Source: CAD feature listing. Evaluate the final solid. Frame: model axes, mm. A direction names the side the tool comes from. Round coordinates to 2 decimals unless told otherwise and drop trailing zeros. Order: outer loops, then holes, each group sorted by start corner. A loop starts at its lowest first (then second) coordinate and runs counter-clockwise, first axis right, second up. Notation, with made-up numbers: (29, 59) -> (68, 59) arc R8 cw to (68, 65) -> close; hole circle Ø10 at (41, 85). An arc over 180 degrees is marked (long way). Write item = value, one per line. Start each with the question number.
(1) Reachability of faces 1 (the face through (13, 2, -26)), 2 (the face through (10, 2, -6)), 3 (the face through (10, 2, -10)) from +Z, -Z, +X, -X, +Y, -Y: full face, straight path, thin tool, end or side. Return the list, or none.
(2) Ray query, line 1 (X direction, y = 1.6, z = -25.25); line 2 (X direction, y = 2.85, z = -17); line 3 (Z direction, x = 9.5, y = 1.35). Return the intervals inside material, ascending.
(3) Cut plane A-A on z = -14.5. Return the cut outline in (x, y), then the cut area to 3 significant figures.
(4) Draft query along X for faces 4 (the face through (16, 2, 0)), 5 (the face through (13, 2, -3)), 6 (the face through (12.703, 2, -16)), 7 (the face through (0, 2, -14)). Return one class per face: released by +X, released by -X, zero draft, split by the parting line, or undercut.
(5) Cut plane B-B on y = 3.05. Return the cut outline in (x, z), then the cut area to 3 significant figures.
from build123d import *

# Parameters (mm, degrees)
SKETCH1_W           = 20
SKETCH1_H           = 28
BOSS_EXTRUDE1_DEPTH = 3.5
SKETCH2_W           = 6
SKETCH2_H           = 4.75
SKETCH2_H_2         = 6
CUT_EXTRUDE1_DEPTH  = 4.5
CUT_EXTRUDE6_DEPTH  = 4.5


with BuildPart() as part:
    # Sketch1 → Boss-Extrude1 (new body)
    with BuildSketch(Plane(origin=(0, 0, 0), x_dir=(1, 0, 0), z_dir=(0, 1, 0))):
        with Locations((10, 14)):
            Rectangle(SKETCH1_W, SKETCH1_H)
    extrude(amount=BOSS_EXTRUDE1_DEPTH)

    # Sketch2 → Cut-Extrude1 (cut, through all)
    with BuildSketch(Plane(origin=(0, 3.5, 0), x_dir=(1, 0, 0), z_dir=(0, 1, 0))):
        with Locations((10, 25.625)):
            Rectangle(SKETCH2_W, SKETCH2_H)
        with Locations((10, 3)):
            Rectangle(SKETCH2_W, SKETCH2_H_2)
    extrude(amount=-CUT_EXTRUDE1_DEPTH, mode=Mode.SUBTRACT)

    # Sketch4 → Cut-Extrude6 (cut, through all)
    with BuildSketch(Plane(origin=(0, 3.5, 0), x_dir=(1, 0, 0), z_dir=(0, 1, 0))):
        with BuildLine():
            Line((12.702975316, 19.34), (12.702975316, 12.66))
            ThreePointArc((12.702975316, 12.66), (10.042975316, 10), (7.382975316, 12.66))
            Line((7.382975316, 12.66), (7.382975316, 19.34))
            ThreePointArc((7.382975316, 19.34), (10.042975316, 22), (12.702975316, 19.34))
        make_face()
    extrude(amount=-CUT_EXTRUDE6_DEPTH, mode=Mode.SUBTRACT)


solid = part.part
Evaluation:
q1.face_1 = -Z, +Y, -Y
q1.face_2 = +Z, +Y, -Y
q1.face_3 = +Y, -Y
q2.line_1 = 0 to 7, 13 to 20
q2.line_2 = 0 to 7.38, 12.7 to 20
q2.line_3 = -23.25 to -21.94, -10.06 to -6
q3.outline = (0, 0) -> (7.38, 0) -> (7.38, 3.5) -> (0, 3.5) -> close; (12.7, 0) -> (20, 0) -> (20, 3.5) -> (12.7, 3.5) -> close
q3.area = 51.4 mm^2
q4.face_4 = zero draft
q4.face_5 = undercut
q4.face_6 = undercut
q4.face_7 = released by -X
q5.outline = (0, -28) -> (7, -28) -> (7, -23.25) -> (13, -23.25) -> (13, -28) -> (20, -28) -> (20, 0) -> (13, 0) -> (13, -6) -> (7, -6) -> (7, 0) -> (0, 0) -> close; hole (7.38, -19.34) arc R2.66 ccw to (12.7, -19.34) -> (12.7, -12.66) arc R2.66 ccw to (7.38, -12.66) -> close
q5.area = 438 mm^2
